Check sheet for the modelled part. Datum: model origin and axes. Units: mm. A direction names the side the tool comes from. Give positions to 0.01 mm unless a question says otherwise; leave off trailing zeros. Write each loop counter-clockwise with the first axis right and the second up, starting at its lowest first coordinate (ties: lowest second). Pieces come first, ordered by that corner, then holes. Notation, with made-up numbers: (-29, 35.25) -> (-23, 35.25) arc R20 ccw to (-23, 54.25) -> close; hole circle Ø9 at (30.5, 61.25). An arc over 180 degrees is marked (long way). Answer as a JSON object with one key per item and string values.
from build123d import *

# Parameters (mm, degrees)
SKETCH1_W           = 9.517416833
SKETCH1_H           = 28.418949141
BOSS_EXTRUDE2_DEPTH = 10
SKETCH4_R           = 1.138899504
CUT_EXTRUDE4_DEPTH  = 10


with BuildPart() as part:
    # Sketch1 → Boss-Extrude2 (new body)
    with BuildSketch(Plane.XY):
        with BuildLine():
            Line((52.348839191, 18.666807499), (52.348839191, 11.781367137))
            ThreePointArc((52.348839191, 11.781367137), (51.636993048, 10.890313034), (50.610732816, 11.387798993))
            Line((50.610732816, 11.387798993), (49.348838236, 14.031369137))
            Line((49.348838236, 14.031369137), (48.348839191, 14.031369137))
            Line((48.348839191, 14.031369137), (48.348839191, -19.226196728))
            ThreePointArc((48.348839191, -19.226196728), (48.061803836, -19.919161373), (47.368839191, -20.206196728))
            Line((47.368839191, -20.206196728), (34.006617177, -20.206196728))
            ThreePointArc((34.006617177, -20.206196728), (33.506618177, -20.706195728), (34.006617177, -21.206194728))
            Line((34.006617177, -21.206194728), (49.531176023, -21.206194728))
            Line((49.531176023, -21.206194728), (49.531176023, -18.353485574))
            ThreePointArc((49.531176023, -18.353485574), (49.672877658, -18.128161546), (49.937346497, -18.158269753))
            Line((49.937346497, -18.158269753), (54.007766524, -21.414600476))
            ThreePointArc((54.007766524, -21.414600476), (54.347138604, -22.597728023), (53.343040178, -23.309592161))
            Line((53.343040178, -23.309592161), (30.246422358, -23.309592161))
            ThreePointArc((30.246422358, -23.309592161), (29.581741984, -23.034272535), (29.306422358, -22.369592161))
            Line((29.306422358, -22.369592161), (29.306422358, 20.294472595))
            ThreePointArc((29.306422358, 20.294472595), (29.581741984, 20.959152969), (30.246422358, 21.234472595))
            Line((30.246422358, 21.234472595), (49.781174095, 21.234472595))
            ThreePointArc((49.781174095, 21.234472595), (51.596787496, 20.4824209), (52.348839191, 18.666807499))
        make_face()
        with Locations((38.827630775, 0.514998025)):
            Rectangle(SKETCH1_W, SKETCH1_H, mode=Mode.SUBTRACT)
    extrude(amount=BOSS_EXTRUDE2_DEPTH)

    # Sketch4 → Cut-Extrude4 (cut)
    with BuildSketch(Plane.ZY.offset(-29.306422358)):
        with Locations((4.548950863, 17.462440217)):
            Circle(SKETCH4_R)
        with Locations((4.551120241, -17.540074349)):
            Circle(SKETCH4_R)
    extrude(amount=-CUT_EXTRUDE4_DEPTH, mode=Mode.SUBTRACT)


solid = part.part
1. Sectioned sample at A-A, the plane x = 40.5. Enter the section's corners in (y, z).
Determined:
{"outline": "(-23.31, 0) -> (-21.21, 0) -> (-21.21, 10) -> (-23.31, 10) -> close; (-20.21, 0) -> (-13.69, 0) -> (-13.69, 10) -> (-20.21, 10) -> close; (14.72, 0) -> (21.23, 0) -> (21.23, 10) -> (14.72, 10) -> close"}
2. Sectioned sample at D-D, the plane z = 8.25. Enter the section's corners in (x, y).
Determined:
{"outline": "(29.31, -22.37) arc R0.94 ccw to (30.25, -23.31) -> (53.34, -23.31) arc R1.06 ccw to (54.01, -21.41) -> (49.94, -18.16) arc R0.25 ccw to (49.53, -18.35) -> (49.53, -21.21) -> (34.01, -21.21) arc R0.5 cw to (34.01, -20.21) -> (47.37, -20.21) arc R0.98 ccw to (48.35, -19.23) -> (48.35, 14.03) -> (49.35, 14.03) -> (50.61, 11.39) arc R0.91 ccw to (52.35, 11.78) -> (52.35, 18.67) arc R2.57 ccw to (49.78, 21.23) -> (30.25, 21.23) arc R0.94 ccw to (29.31, 20.29) -> close; hole (34.07, -13.69) -> (43.59, -13.69) -> (43.59, 14.72) -> (34.07, 14.72) -> close"}
3. Access from +Z, -Z, +X, -X, +Y, -Y to the whole of each face (thin tool, end or side, straight path). Record for faces 4 (the face through (34.24, -18.55, 5.08)), 5 (the face through (33.507, -20.695, 4.93)), 6 (the face through (51.94, -19.76, 4.93)).
Determined:
{"face 4": "-X", "face 5": "+Z, -Z", "face 6": "+Z, -Z, +X"}
4. Scan lines: L1, parallel to Y at x = 40.75, z = 8.5; L2, parallel to X at y = -11, z = 9.75; L3, parallel to Y at x = 38.75, z = 4.25. Record each from-to range of solid material in increasing order. Write a range as [from, to].
Determined:
{"L1": "[-23.31, -21.21], [-20.21, -13.69], [14.72, 21.23]", "L2": "[29.31, 34.07], [43.59, 48.35]", "L3": "[-23.31, -21.21], [-20.21, -18.64], [-16.44, -13.69], [14.72, 16.36], [18.56, 21.23]"}
5. Sectioned sample at B-B, the plane y = 8. Enter the section's corners in (x, z), plus the area to 4 significant figures.
Determined:
{"outline": "(29.31, 0) -> (34.07, 0) -> (34.07, 10) -> (29.31, 10) -> close; (43.59, 0) -> (48.35, 0) -> (48.35, 10) -> (43.59, 10) -> close", "area": "95.25 mm^2"}
6. Sectioned sample at C-C, the plane x = 46. Enter the section's corners in (y, z), plus the area to 3 significant figures.
Determined:
{"outline": "(-23.31, 0) -> (-21.21, 0) -> (-21.21, 10) -> (-23.31, 10) -> close; (-20.21, 0) -> (21.23, 0) -> (21.23, 10) -> (-20.21, 10) -> close", "area": "435 mm^2"}
7. Mould release check, pull along X, two halves, no side actions. Record for faces 1 (the face through (41, -20.206, 5)), 2 (the face through (34.24, 16.35, 4.3)), 3 (the face through (51.58, 20.5, 4.93)): released by +X, released by -X, zero draft, split by the parting line, or undercut.
Determined:
{"face 1": "undercut", "face 2": "zero draft", "face 3": "released by +X"}
8. Go/stop test with flat-tipped pins: P1, Ø1, axis at y = 5.5, z = 7.5, coming from the +X side; P2, Ø3.5, axis at y = 17.46, z = 4.55, coming from the +X side; P3, Ø2, axis at y = -17.54, z = 4.55, coming from the +X side. Record where each tip stops, or that it passes through.
Determined:
{"P1": "x = 48.35", "P2": "x = 52.35", "P3": "x = 50.41"}
